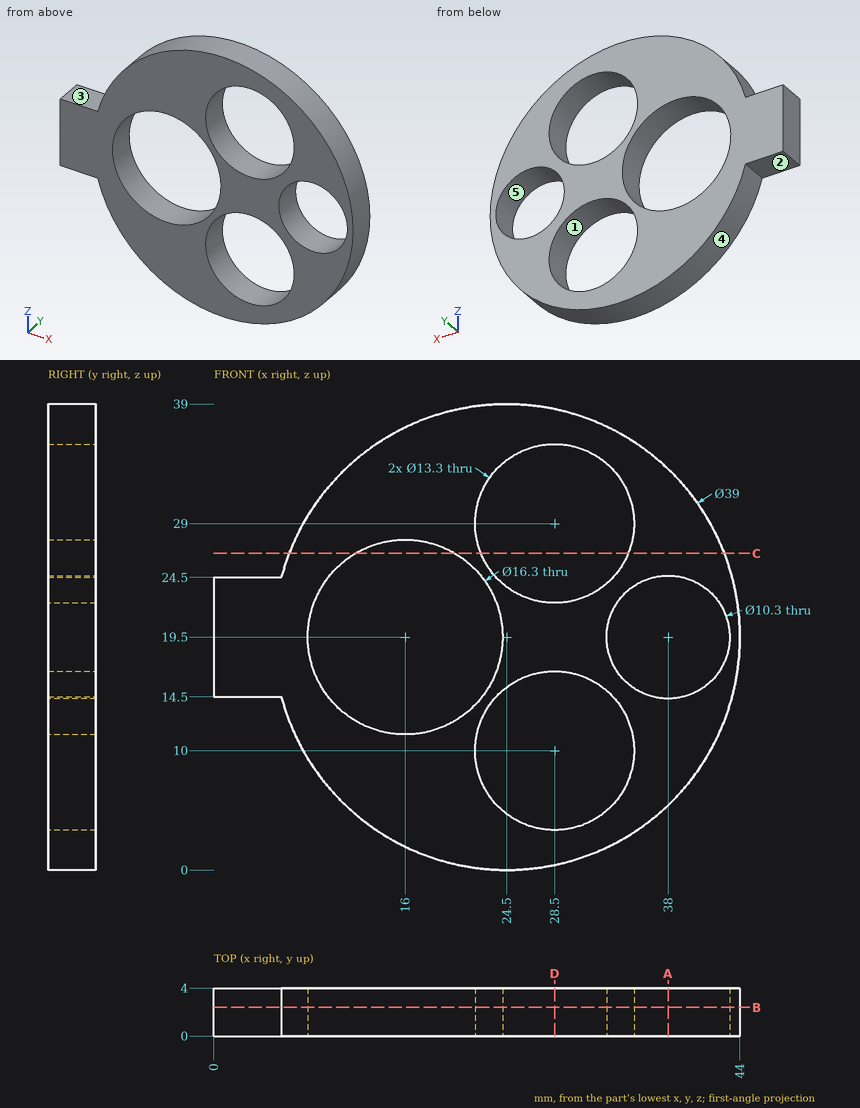
Study the drawing (mm; zero at the part's minimum x, y, z) and answer. A direction names the side the tool comes from. Coordinates: 2 decimals unless noted, no trailing zeros. Loops run counter-clockwise (first coordinate to the right, second up) from the corner with the lowest first, then second, coordinate; pieces in that order, holes last. Notation, with made-up numbers: (70, 53.25) -> (81, 53.25) arc R15 cw to (81, 71.25) -> close; hole circle Ø3 at (43, -36). An arc over 180 degrees is marked (long way). Write each question's results on one line, items separated by ' | '. Start each with the question number.
1) Consider line 1 along X through (y, z) = (2.8, 13); line 2 along Z through (x, y) = (32.5, 1.35); line 3 along Z through (x, y) = (4, 0.4). Determine where each line is inside the solid, lowest interval first.
2) Find section B-B on y = 2.4. Determine the outline of the cut face in (x, z), then the cut area to 3 significant figures.
3) Find section D-D on x = 28.5. Determine the outline of the cut face in (y, z).
4) Find section C-C on z = 26.5. Determine the outline of the cut face in (x, y), then the cut area to 3 significant figures.
5) Flat-ended cylindrical pins translate along their axes: P1, Ø1.2, axis at x = 4, y = 1.5, coming from the +Z side; P2, Ø2, axis at x = 3.5, y = 2, coming from the -Z side; P3, Ø2, axis at x = 19, y = 1.5, coming from the +Z side. Find the tip coordinate at first contact, or state that the pin passes through.
6) The mould has two halves that part along Z. Classify the marked faces 3, 4 and 5: pulls with the +Z half, pulls with the -Z half, needs draft (parallel to the pull), parting line crosses it, or undercut.
7) Find section A-A on x = 38. Determine the outline of the cut face in (y, z).
8) For the marked faces 1 and 2, determine the directions among +Z, -Z, +X, -X, +Y, -Y from which every point of the face is accessible in a straight line to the end or side of a thin tool.
Response values:
1) line 1: x = 6.12 to 11.08, 20.92 to 22.57, 34.43 to 42.88 | line 2: z = 1.72 to 4.69, 15.31 to 23.69, 34.31 to 37.28 | line 3: z = 14.5 to 24.5
2) outline: (0, 14.5) -> (5.65, 14.5) arc R19.5 ccw (long way) to (5.65, 24.5) -> (0, 24.5) -> close; hole circle Ø16.3 at (16, 19.5); hole circle Ø13.3 at (28.5, 10); hole circle Ø13.3 at (28.5, 29); hole circle Ø10.3 at (38, 19.5) | area: 677 mm^2
3) outline: (0, 0.41) -> (4, 0.41) -> (4, 3.35) -> (0, 3.35) -> close; (0, 16.65) -> (4, 16.65) -> (4, 22.35) -> (0, 22.35) -> close; (0, 35.65) -> (4, 35.65) -> (4, 38.59) -> (0, 38.59) -> close
4) outline: (6.3, 0) -> (11.83, 0) -> (11.83, 4) -> (6.3, 4) -> close; (20.17, 0) -> (22.34, 0) -> (22.34, 4) -> (20.17, 4) -> close; (34.66, 0) -> (42.7, 0) -> (42.7, 4) -> (34.66, 4) -> close | area: 62.9 mm^2
5) P1: stops at z = 24.5 | P2: stops at z = 14.5 | P3: stops at z = 38.47
6) face 3: pulls with the +Z half | face 4: parting line crosses it | face 5: undercut
7) outline: (0, 5.43) -> (4, 5.43) -> (4, 14.35) -> (0, 14.35) -> close; (0, 24.65) -> (4, 24.65) -> (4, 33.57) -> (0, 33.57) -> close
8) face 1: +Y, -Y | face 2: -Z, -X, +Y, -Y
